Check sheet for the modelled part. Datum: model origin and axes. Units: mm. Coordinates: 2 decimals unless noted, no trailing zeros. Order: outer loops, then holes, each group sorted by start corner. A loop starts at its lowest first (then second) coordinate and runs counter-clockwise, first axis right, second up.
from build123d import *

# Parameters (mm, degrees)
SKETCH1_W           = 568.96
SKETCH1_H           = 568.96
BOSS_EXTRUDE1_DEPTH = 3.175
SKETCH3_R           = 12.5
SKETCH3_R_2         = 1.55
SKETCH3_R_3         = 2.55
CUT_EXTRUDE2_DEPTH  = 6.35
SKETCH4_R           = 2.55
SKETCH4_W           = 505.46
SKETCH4_H           = 441.96
CUT_EXTRUDE4_DEPTH  = 6.35
CHAMFER1_SIZE       = 3.2


with BuildPart() as part:
    # Sketch1 → Boss-Extrude1 (new, symmetric)
    with BuildSketch(Plane(origin=(0, 0, 0), x_dir=(1, 0, 0), z_dir=(0, 1, 0))):
        Rectangle(SKETCH1_W, SKETCH1_H)
    extrude(amount=BOSS_EXTRUDE1_DEPTH, both=True)

    # Sketch3 → Cut-Extrude2 (cut)
    with BuildSketch(Plane(origin=(0, 3.175, 0), x_dir=(1, 0, 0), z_dir=(0, 1, 0))):
        with Locations(Location((-244.475, 259.4, 0), (0, 0, 270))):
            Circle(SKETCH3_R)
        with Locations(Location((-259.969, 274.4, 0), (0, 0, 270))):
            Circle(SKETCH3_R_2)
        with Locations(Location((-228.981, 274.399982938, 0), (0, 0, 270))):
            Circle(SKETCH3_R_2)
        with Locations(Location((-228.981017062, 243.411982938, 0), (0, 0, 270))):
            Circle(SKETCH3_R_2)
        with Locations(Location((-259.969017062, 243.412, 0), (0, 0, 270))):
            Circle(SKETCH3_R_2)
        with Locations(Location((-244.475, -268.605, 0), (0, 0, 270))):
            Circle(SKETCH3_R_3)
    cut_extrude2 = extrude(amount=-CUT_EXTRUDE2_DEPTH, mode=Mode.SUBTRACT)

    # Mirror2: Cut-Extrude2 across plane
    add(cut_extrude2.mirror(Plane(origin=(0, 0, 0), x_dir=(0, 0, 1), z_dir=(1, 0, 0))), mode=Mode.SUBTRACT)

    # Sketch4 → Cut-Extrude4 (cut)
    with BuildSketch(Plane(origin=(0, 3.175, 0), x_dir=(1, 0, 0), z_dir=(0, 1, 0))):
        with Locations(Location((-225.425, 215.42375, 0), (0, 0, 270))):
            Circle(SKETCH4_R)
        with Locations(Location((-263.525, 215.42375, 0), (0, 0, 90))):
            Circle(SKETCH4_R)
        with Locations(Location((-263.525, 229.64775, 0), (0, 0, 90))):
            Circle(SKETCH4_R)
        with Locations(Location((-225.425, 229.64775, 0), (0, 0, 270))):
            Circle(SKETCH4_R)
        with Locations(Location((263.525, 229.64775, 0), (0, 0, 270))):
            Circle(SKETCH4_R)
        with Locations(Location((263.525, 215.42375, 0), (0, 0, 270))):
            Circle(SKETCH4_R)
        with Locations(Location((225.425, 215.42375, 0), (0, 0, 90))):
            Circle(SKETCH4_R)
        with Locations(Location((225.425, 229.64775, 0), (0, 0, 90))):
            Circle(SKETCH4_R)
        with Locations(Location((225.425, -240.82375, 0), (0, 0, 270))):
            Circle(SKETCH4_R)
        with Locations(Location((225.425, -255.04775, 0), (0, 0, 270))):
            Circle(SKETCH4_R)
        with Locations(Location((263.525, -240.82375, 0), (0, 0, 90))):
            Circle(SKETCH4_R)
        with Locations(Location((263.525, -255.04775, 0), (0, 0, 90))):
            Circle(SKETCH4_R)
        with Locations(Location((-225.425, -240.82375, 0), (0, 0, 90))):
            Circle(SKETCH4_R)
        with Locations(Location((-263.525, -240.82375, 0), (0, 0, 270))):
            Circle(SKETCH4_R)
        with Locations(Location((-225.425, -255.04775, 0), (0, 0, 90))):
            Circle(SKETCH4_R)
        with Locations(Location((-263.525, -255.04775, 0), (0, 0, 270))):
            Circle(SKETCH4_R)
        with Locations((0, -12.7)):
            Rectangle(SKETCH4_W, SKETCH4_H)
    extrude(amount=-CUT_EXTRUDE4_DEPTH, mode=Mode.SUBTRACT)

    # Chamfer1
    chamfer1_edges = [part.edges().sort_by_distance(p)[0] for p in [
        (225.425, 3.175, -212.87375),
        (225.425, 3.175, -227.09775),
        (225.425, 3.175, 238.27375),
        (225.425, 3.175, 252.49775),
        (263.525, 3.175, 243.37375),
        (263.525, 3.175, 257.59775),
        (-225.425, 3.175, 243.37375),
        (-263.525, 3.175, 238.27375),
        (-225.425, 3.175, 257.59775),
        (-263.525, 3.175, 252.49775),
        (-225.425, 3.175, -217.97375),
        (-263.525, 3.175, -212.87375),
        (-225.425, 3.175, -232.19775),
        (-263.525, 3.175, -227.09775),
        (263.525, 3.175, -232.19775),
        (263.525, 3.175, -217.97375),
    ]]
    chamfer(chamfer1_edges, length=CHAMFER1_SIZE)


solid = part.part
(1) Cross-section at B-B (x = -23.5). Enter the section's corners in (y, z) (3 decimals).
Filled in:
outline: (-3.175, -284.48) - (3.175, -284.48) - (3.175, -208.28) - (-3.175, -208.28) - close; (-3.175, 233.68) - (3.175, 233.68) - (3.175, 284.48) - (-3.175, 284.48) - close
(2) Cross-section at D-D (y = 1.75). Count the separate pieces of the cut face and the enclosed holes in it, and give its area (3 significant figures).
Filled in:
separate pieces: 1
enclosed holes: 29
area: 98,300 mm2
(3) Cross-section at A-A (z = -259.4). Enter the section's corners in (x, y) (3 decimals).
Filled in:
outline: (-284.48, -3.175) - (-256.975, -3.175) - (-256.975, 3.175) - (-284.48, 3.175) - close; (-231.975, -3.175) - (231.975, -3.175) - (231.975, 3.175) - (-231.975, 3.175) - close; (256.975, -3.175) - (284.48, -3.175) - (284.48, 3.175) - (256.975, 3.175) - close
(4) Cross-section at C-C (z = 139). Enter the section's corners in (x, y) (3 decimals), and give its area (3 significant figures).
Filled in:
outline: (-284.48, -3.175) - (-252.73, -3.175) - (-252.73, 3.175) - (-284.48, 3.175) - close; (252.73, -3.175) - (284.48, -3.175) - (284.48, 3.175) - (252.73, 3.175) - close
area: 403 mm2
(5) Go/stop test with flat-tipped pins: P1, Ø4, axis at x = 244.475, z = 268.605, coming from the +Y side; P2, Ø6, axis at x = -225.42, z = -229.65, coming from the +Y side. Record where each tip stops, or that it passes through.
Filled in:
P1: passes through
P2: stops at y = 0.43
(6) Thickness scan on probe 1 along X at (y, z) = (0.75, 25); probe 2 along Z at (x, y) = (-25, -1.25); probe 3 along X at (y, z) = (2.5, 252.5). Record the ranges inside material, lowest first.
Filled in:
probe 1: x = -284.48 to -252.73, 252.73 to 284.48
probe 2: z = -284.48 to -208.28, 233.68 to 284.48
probe 3: x = -284.48 to -267.91, -259.14 to -229.81, -221.04 to 221.04, 229.81 to 259.14, 267.91 to 284.48
(7) Release check for a two-part mould opening along X. For faces 1 (the flat face through (-22, 3.175, -212)), 2 (the cylindrical face through (255.565, 0.044, -253.632)) record: +X half, -X half, draft (parallel to the pull), parting line (faces both ways), or undercut.
Filled in:
face 1: draft
face 2: undercut
